Autodesk Inventor part; units mm, degrees
ref_plane "YZ Plane" through (0, 0, 0) normal (1, 0, 0) x (0, 1, 0)
ref_plane "XZ Plane" through (0, 0, 0) normal (0, 1, 0) x (-1, 0, 0)
ref_plane "XY Plane" through (0, 0, 0) normal (0, 0, 1) x (1, 0, 0)
sketch "Sketch1" plane through (0, 0, 0) normal (0, 0, 1) x (1, 0, 0)
  line L0 (0, 0) -> (5, 0)
  line L1 (5, 0) -> (5, 20)
  line L2 (5, 20) -> (0, 20)
  line L3 (0, 20) -> (0, 0)
  dimension "d0" = 5
  dimension "d1" = 20
extrude "Extrusion1" add sketch "Sketch1" along normal blind 15
sketch "Sketch2" plane through (0, 0, 15) normal (0, 0, 1) x (1, 0, 0)
  line L0 (5, 20) -> (0, 20)
  circle A0 centre (2.5, 3) radius 1.5
  line L1 (0, 20) -> (0, 0)
  line L2 (0, 10) -> (5, 10)
  line L3 (5, 0) -> (5, 20)
  circle A1 centre (2.5, 17) radius 1.5
  line L4 (0, 0) -> (5, 0)
  point P0 (2.5, 0)
  dimension "d4" = 3
  dimension "d12" = 3
hole "Hole1" at (2.5, 17, 15) at (2.5, 3, 15) direction (0, 0, -1) diameter 2.459 end through all
sketch "Sketch3" plane through (0, 0, 15) normal (0, 0, 1) x (1, 0, 0)
  line L0 (0, 20) -> (0, 0)
  line L1 (0, 10) -> (5, 10)
  line L2 (5, 0) -> (5, 20)
sketch "Sketch6" plane through (0, 0, 0) normal (-1, 0, 0) x (0, 0, 1)
  line L0 (0, 0) -> (0, 20)
  line L1 (0, 0) -> (15, 0)
  line L2 (15, 0) -> (15, -20)
  line L3 (15, -20) -> (0, -20)
  line L4 (0, -20) -> (0, 0)
  dimension "d24" = 15
  dimension "d25" = 20
extrude "Extrusion2" add sketch "Sketch6" against normal blind 5
sketch "Sketch9" plane through (0, 20, 0) normal (-1, 0, 0) x (0, 0, 1)
  line L0 (0, -20) -> (15, -20)
  line L1 (15, 0) -> (15, -40)
  circle A0 centre (5, -35) radius 2.5
  line L2 (0, -40) -> (15, -40)
  line L3 (0, 0) -> (0, -40)
  point P0 (7.5, -40)
  dimension "d28" = 5
  dimension "d37" = 5
  dimension "d38" = 5
hole "Hole3" at (0, -15, 5) direction (1, 0, 0) diameter 4.5 end through all
properties part number "Al Attach block"
The listing builds one solid part. Answer for the finished solid, in the listing's coordinates (mm). Coordinates: 2 decimals unless noted, no trailing zeros. Write each loop counter-clockwise with the first axis right and the second up, starting at its lowest first coordinate (ties: lowest second). Pieces come first, ordered by that corner, then holes.
Q1. Section C-C, the plane x = 2.1 is taken. Write down the section's boundary in (y, z), then the cut area to 3 significant figures.
Returned:
outline: (-20, 0) - (1.84, 0) - (1.84, 15) - (-20, 15) - close; (4.16, 0) - (15.84, 0) - (15.84, 15) - (4.16, 15) - close; (18.16, 0) - (20, 0) - (20, 15) - (18.16, 15) - close; hole circle Ø4.5 at (-15, 5)
area: 514 mm2
Q2. Section B-B, the plane y = -15 is taken. Write down the section's boundary in (x, z), then the cut area to 3 significant figures.
Returned:
outline: (0, 0) - (5, 0) - (5, 2.75) - (0, 2.75) - close; (0, 7.25) - (5, 7.25) - (5, 15) - (0, 15) - close
area: 52.5 mm2
Q3. Section D-D, the plane z = 10 is taken. Write down the section's boundary in (x, y), then the cut area to 3 significant figures.
Returned:
outline: (0, -20) - (5, -20) - (5, 20) - (0, 20) - close; hole circle Ø2.46 at (2.5, 3); hole circle Ø2.46 at (2.5, 17)
area: 191 mm2
Q4. The mould has two halves that part along Y. Classify faces 1 (the flat face through (2, 0, 15)), 2 (the cylindrical face through (2.131, 15.827, 7.395)), 3 (the flat face through (2, -20, 8)): released by +Y, released by -Y, zero draft, split by the parting line, or undercut.
Returned:
face 1: zero draft
face 2: undercut
face 3: released by -Y
Q5. Find the intervals of material crossed by line 1 along X through (y, z) = (3, 9.25); line 2 along Y through (x, z) = (2.25, 14.25); line 3 along Y through (x, z) = (2.6, 4.5), in increasing order.
Returned:
line 1: x = 0 to 1.27, 3.73 to 5
line 2: y = -20 to 1.8, 4.2 to 15.8, 18.2 to 20
line 3: y = -20 to -17.19, -12.81 to 1.77, 4.23 to 15.77, 18.23 to 20
Q6. Given P1, Ø2, axis at x = 2.5, y = 3, coming from the -Z side, flat-ended and moving along its own axis, determine where the tip first touches the part or whether it passes through.
Returned:
P1: passes through
Q7. Section A-A, the plane z = 5 is taken. Write down the section's boundary in (x, y).
Returned:
outline: (0, -20) - (5, -20) - (5, -17.25) - (0, -17.25) - close; (0, -12.75) - (5, -12.75) - (5, 20) - (0, 20) - close; hole circle Ø2.46 at (2.5, 3); hole circle Ø2.46 at (2.5, 17)
